from build123d import *

# Parameters (mm, degrees)
SKETCH1_R                      = 16.51
SKETCH1_R_2                    = 13.97
BOSS_EXTRUDE1_DEPTH            = 22.225
BOSS_EXTRUDE2_START            = 4.7625
SKETCH1_2_R                    = 16.51
BOSS_EXTRUDE2_DEPTH            = 4.7625
F_5_16_0_3125_DIAMETER_HOLE1_D = 7.9375


with BuildPart() as part:
    # Sketch1 → Boss-Extrude1 (new body)
    with BuildSketch(Plane(origin=(0, 0, 0), x_dir=(1, 0, 0), z_dir=(0, 1, 0))):
        with Locations(Location((0, 0, 0), (0, 0, 270))):
            Circle(SKETCH1_R)
        with Locations(Location((0, 0, 0), (0, 0, 270))):
            Circle(SKETCH1_R_2, mode=Mode.SUBTRACT)
    extrude(amount=-BOSS_EXTRUDE1_DEPTH)

    # Sketch1<2> → Boss-Extrude2 (add)
    with BuildSketch(Plane(origin=(0, 0, 0), x_dir=(1, 0, 0), z_dir=(0, 1, 0)).offset(BOSS_EXTRUDE2_START)):
        with Locations(Location((0, 0, 0), (0, 0, 270))):
            Circle(SKETCH1_2_R)
    extrude(amount=-BOSS_EXTRUDE2_DEPTH)

    # 5/16 (0.3125) Diameter Hole1 (through all)
    with Locations(Plane(origin=(0, 4.7625, 0), x_dir=(1, 0, 0), z_dir=(0, 1, 0))):
        with Locations((0, 0)):
            Hole(F_5_16_0_3125_DIAMETER_HOLE1_D / 2)


solid = part.part
Build history of the part. All positions in model axes, mm. A direction names the side the tool comes from. Give positions to 0.01 mm unless a question says otherwise; leave off trailing zeros. Order: outer loops, then holes, each group sorted by start corner. A loop starts at its lowest first (then second) coordinate and runs counter-clockwise, first axis right, second up. Notation, with made-up numbers: M -29,83.5 L -15,83.5 A26 cw -15,112.5 Z; hole C 58.5,-34.75 d8. An arc over 180 degrees is marked long. Put each result on its own line as item: value.
Item 1: Slice it at D-D, the plane z = -6.5. Write the cut outline in (x, y) (1 decimal).
From the geometry:
outline: M -15.2,-22.2 L -12.4,-22.2 L -12.4,0 L 12.4,0 L 12.4,-22.2 L 15.2,-22.2 L 15.2,4.8 L -15.2,4.8 Z
Item 2: 3-axis set-ups, long thin cutter, end or side, ignore diameter. For faces 4 (the cylindrical face through (13.85, -10.96, -1.82)), 5 (the flat face through (-3, 4.762, 3)): which of +Z, -Z, +X, -X, +Y, -Y reach the whole face in a straight line?
From the geometry:
face 4: -Y
face 5: +Z, -Z, +X, -X, +Y
Item 3: Slice it at B-B, the plane x = 0. Write the cut outline in (y, z) (1 decimal), plus the area to 3 significant figures.
From the geometry:
outline: M -22.2,-16.5 L 4.8,-16.5 L 4.8,-4 L 0,-4 L 0,-14 L -22.2,-14 Z; M -22.2,14 L 0,14 L 0,4 L 4.8,4 L 4.8,16.5 L -22.2,16.5 Z
area: 232 mm2
Item 4: Flat gauge pins, fed straight in: pin 1 Ø3 at (x, y) = (-3.5, -6.5) entering from -Z; pin 2 Ø10 at (y, z) = (-11.5, -5) entering from -X; pin 3 Ø1.5 at (y, z) = (-15, -8.5) entering from -X; pin 4 Ø3 at (x, z) = (-1, -1.5) entering from +Y. Where does each tip first touch, or does it go through?
From the geometry:
pin 1: stops at z = -16.39
pin 2: stops at x = -16.51
pin 3: stops at x = -14.58
pin 4: passes through
Item 5: Probe line 1 (Y direction, x = -6, z = -4); line 2 (X direction, y = -13.5, z = -0.5); line 3 (X direction, y = -14.25, z = -8.5). List the from-to ranges inside material, lowest first. Write a range as [from, to].
From the geometry:
line 1: y = [0, 4.76]
line 2: x = [-16.5, -13.96], [13.96, 16.5]
line 3: x = [-14.15, -11.09], [11.09, 14.15]
Item 6: Two-plate mould, pull along X, no slides. Class faces 1 (the cylindrical face through (-10.05, -8.54, -13.1)), 2 (the flat face through (4, -22.225, -14)), 3 (the flat face through (-3, 0, 3)): +X half, -X half, draft (parallel to the pull), parting line (faces both ways), or undercut.
From the geometry:
face 1: parting line
face 2: draft
face 3: undercut
Item 7: Slice it at A-A, the plane z = 0. Write the cut outline in (x, y) (1 decimal), plus the area to 3 significant figures.
From the geometry:
outline: M -16.5,-22.2 L -14,-22.2 L -14,0 L -4,0 L -4,4.8 L -16.5,4.8 Z; M 4,0 L 14,0 L 14,-22.2 L 16.5,-22.2 L 16.5,4.8 L 4,4.8 Z
area: 232 mm2
Item 8: Slice it at C-C, the plane y = -16. Write the cut outline in (x, z).
From the geometry:
outline: C 0,0 d33.02; hole C 0,0 d27.94
